Check sheet for the drawn part. Datum: minimum x, y, z corner. Units: mm. Round coordinates to 2 decimals unless told otherwise and drop trailing zeros. Loops run counter-clockwise (first coordinate to the right, second up) from the corner with the lowest first, then second, coordinate; pieces in that order, holes last.
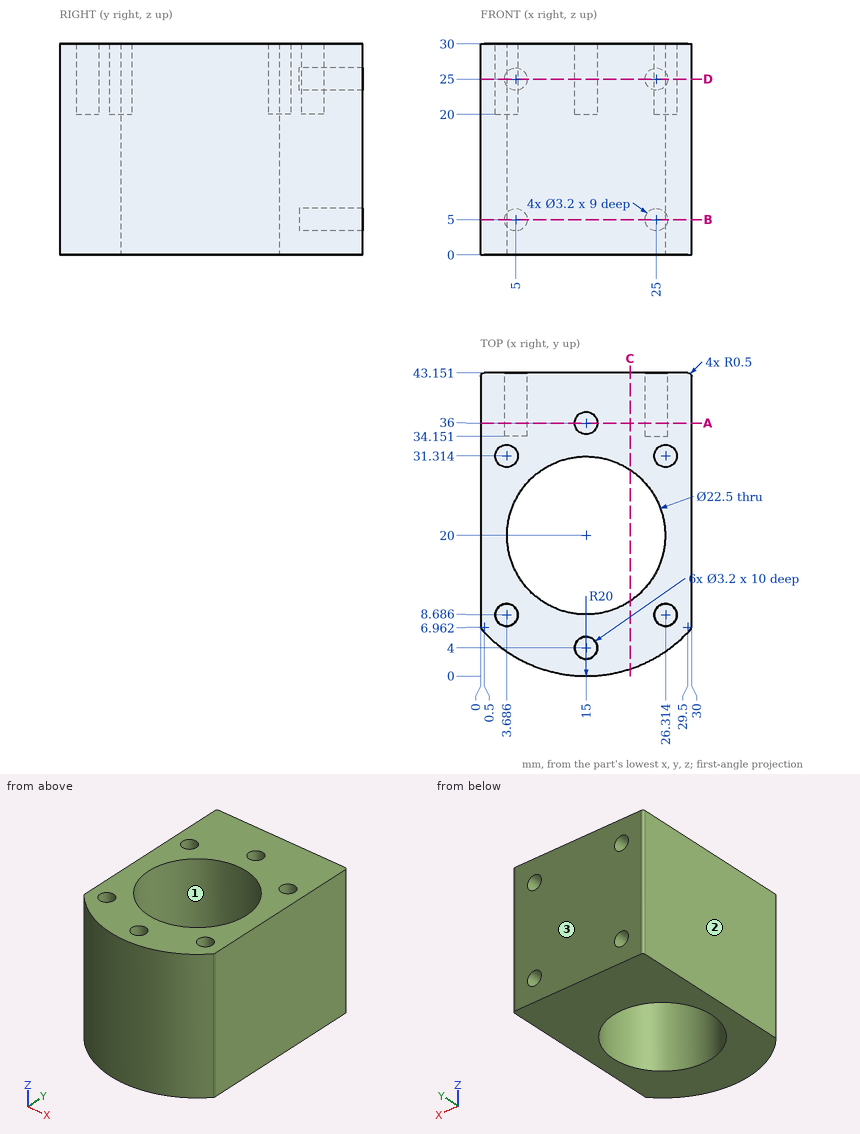
1) Mould release check, pull along Y, two halves, no side actions. Record for the marked faces 1, 2 and 3: +Y half, -Y half, draft (parallel to the pull), parting line (faces both ways), or undercut.
Report:
face 1: undercut
face 2: draft
face 3: +Y half
2) Sectioned sample at B-B, the plane z = 5. Record the cut outline in (x, y).
Report:
outline: (0, 6.96) arc R0.5 ccw to (0.13, 6.63) arc R20 ccw to (29.87, 6.63) arc R0.5 ccw to (30, 6.96) - (30, 42.65) arc R0.5 ccw to (29.5, 43.15) - (26.6, 43.15) - (26.6, 34.15) - (23.4, 34.15) - (23.4, 43.15) - (6.6, 43.15) - (6.6, 34.15) - (3.4, 34.15) - (3.4, 43.15) - (0.5, 43.15) arc R0.5 ccw to (0, 42.65) - close; hole circle Ø22.5 at (15, 20)
3) Sectioned sample at D-D, the plane z = 25. Record the cut outline in (x, y).
Report:
outline: (0, 6.96) arc R0.5 ccw to (0.13, 6.63) arc R20 ccw to (29.87, 6.63) arc R0.5 ccw to (30, 6.96) - (30, 42.65) arc R0.5 ccw to (29.5, 43.15) - (26.6, 43.15) - (26.6, 34.15) - (23.4, 34.15) - (23.4, 43.15) - (6.6, 43.15) - (6.6, 34.15) - (3.4, 34.15) - (3.4, 43.15) - (0.5, 43.15) arc R0.5 ccw to (0, 42.65) - close; hole circle Ø3.2 at (3.69, 8.69); hole circle Ø3.2 at (3.69, 31.31); hole circle Ø22.5 at (15, 20); hole circle Ø3.2 at (15, 4); hole circle Ø3.2 at (15, 36); hole circle Ø3.2 at (26.31, 8.69); hole circle Ø3.2 at (26.31, 31.31)
4) Gauge pin test, flat ends, axial feed: pin 1 (1.9 mm diameter, centred on x = 5, z = 5, fed in from +Y); pin 2 (1.9 mm diameter, centred on x = 3.69, y = 8.69, fed in from +Z); pin 3 (1.5 mm diameter, centred on x = 4.5, z = 26.5, fed in from -Y). Record the tip position at first contact, or that the pin passes through.
Report:
pin 1: stops at y = 34.15
pin 2: stops at z = 20
pin 3: stops at y = 2.54
5) Scan lines: line 1 along X through (y, z) = (38, 25); line 2 along X through (y, z) = (32.5, 24.5) (1 decimal); line 3 along Y through (x, z) = (15.25, 28). Record each from-to range of solid material in increasing order.
Report:
line 1: x = 0 to 3.4, 6.6 to 23.4, 26.6 to 30
line 2: x = 0 to 2.6, 4.8 to 25.2, 27.4 to 30
line 3: y = 0 to 2.42, 5.58 to 8.75, 31.25 to 34.42, 37.58 to 43.15
6) Sectioned sample at A-A, the plane y = 36. Record the cut outline in (x, z).
Report:
outline: (0, 0) - (30, 0) - (30, 30) - (16.6, 30) - (16.6, 20) - (13.4, 20) - (13.4, 30) - (0, 30) - close; hole circle Ø3.2 at (5, 5); hole circle Ø3.2 at (5, 25); hole circle Ø3.2 at (25, 5); hole circle Ø3.2 at (25, 25)
7) Sectioned sample at C-C, the plane x = 21.25. Record the cut outline in (y, z), then the cut area to 3 significant figures.
Report:
outline: (1, 0) - (10.65, 0) - (10.65, 30) - (1, 30) - close; (29.35, 0) - (43.15, 0) - (43.15, 30) - (29.35, 30) - close
area: 703 mm2
